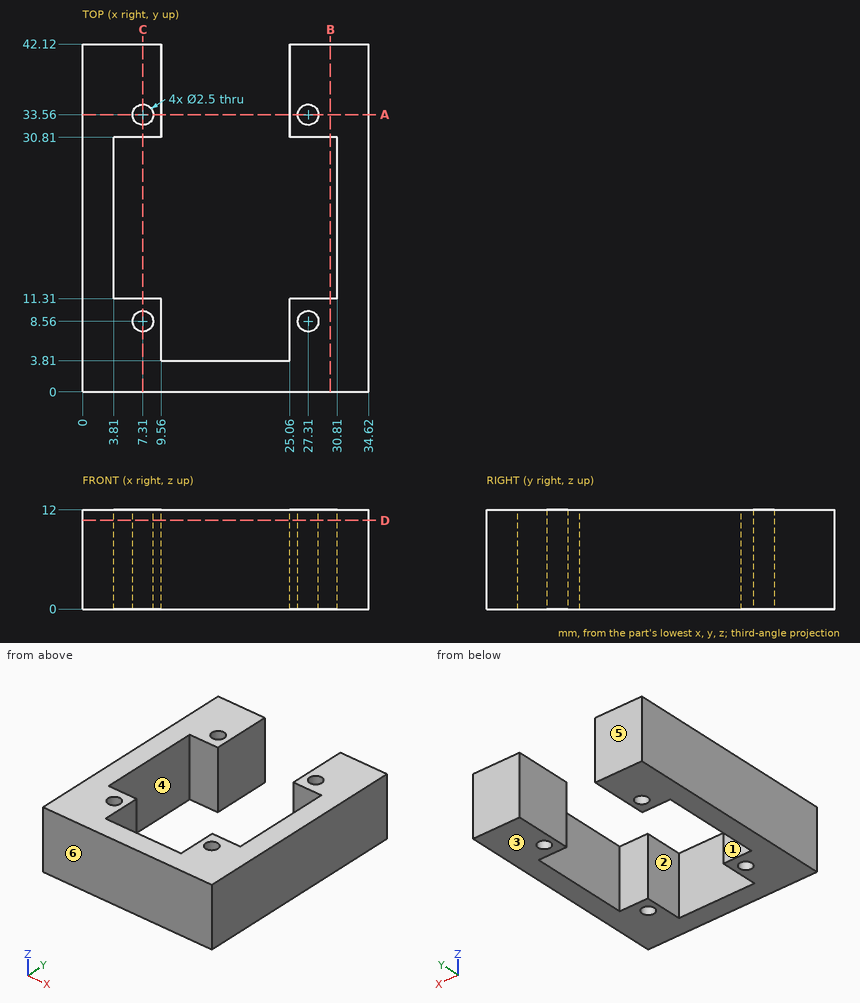
Input: dimensioned drawing with shaded views. Units: mm. Origin: part minimum x, y, z. A direction names the side the tool comes from. Coordinates: 2 decimals unless noted, no trailing zeros. Write each loop counter-clockwise with the first axis right and the second up, starting at its lowest first coordinate (ties: lowest second). Pieces come first, ordered by that corner, then holes. Notation, with made-up numbers: M 55,47 L 67,47 A28 ccw 67,84 Z; hole C 56,57.5 d3. An arc over 180 degrees is marked long. Use one line per item in the form item = value.
Q1. Material intervals for probe 1 along X at (y, z) = (33.56, 3.75); probe 2 along Y at (x, z) = (7.31, 7.5); probe 3 along Y at (x, z) = (25.5, 1.75), sorted ascending. Write a range as from..to.
Answer below:
probe_1 = 0..6.06, 8.56..9.56, 25.06..26.06, 28.56..34.62
probe_2 = 0..7.31, 9.81..11.31, 30.81..32.31, 34.81..42.12
probe_3 = 0..11.31, 30.81..42.12
Q2. Set-up query: the marked faces 1, 2 and 3. Return all of +Z, -Z, +X, -X, +Y, -Y with unobstructed straight access to the full face (end or side cutting, diameter ignored); none if empty.
Answer below:
face_1 = +Z, -Z
face_2 = +Z, -Z, +Y
face_3 = -Z, +X, -X, +Y, -Y
Q3. Section B-B (x = 30). Return loops of the section in (y, z), plus the area to 3 significant figures.
Answer below:
outline = M 0,0 L 11.31,0 L 11.31,12 L 0,12 Z; M 30.81,0 L 42.12,0 L 42.12,12 L 30.81,12 Z
area = 271 mm²
Q4. Section D-D (z = 10.75). Return loops of the section in (x, y).
Answer below:
outline = M 0,0 L 34.62,0 L 34.62,42.12 L 25.06,42.12 L 25.06,30.81 L 30.81,30.81 L 30.81,11.31 L 25.06,11.31 L 25.06,3.81 L 9.56,3.81 L 9.56,11.31 L 3.81,11.31 L 3.81,30.81 L 9.56,30.81 L 9.56,42.12 L 0,42.12 Z; hole C 7.31,8.56 d2.5; hole C 7.31,33.56 d2.5; hole C 27.31,8.56 d2.5; hole C 27.31,33.56 d2.5
Q5. Section C-C (x = 7.31). Return loops of the section in (y, z).
Answer below:
outline = M 0,0 L 7.31,0 L 7.31,12 L 0,12 Z; M 9.81,0 L 11.31,0 L 11.31,12 L 9.81,12 Z; M 30.81,0 L 32.31,0 L 32.31,12 L 30.81,12 Z; M 34.81,0 L 42.12,0 L 42.12,12 L 34.81,12 Z
Q6. Section A-A (y = 33.56). Return loops of the section in (x, z), plus the area to 3 significant figures.
Answer below:
outline = M 0,0 L 6.06,0 L 6.06,12 L 0,12 Z; M 8.56,0 L 9.56,0 L 9.56,12 L 8.56,12 Z; M 25.06,0 L 26.06,0 L 26.06,12 L 25.06,12 Z; M 28.56,0 L 34.62,0 L 34.62,12 L 28.56,12 Z
area = 169 mm²
Q7. Draft query along Y for the marked faces 4, 5 and 6. Return one class per face: released by +Y, released by -Y, zero draft, split by the parting line, or undercut.
Answer below:
face_4 = undercut
face_5 = released by +Y
face_6 = released by -Y
Q8. First-contact query: pin 1 (3.5 mm diameter, centred on x = 19.5, z = 6, fed in from +Y). Flat tip, straight axial feed; report the tip coordinate or a pass-through.
Answer below:
pin_1 = 3.81
